Verification items for this drawing (mm, ordinates from the low corner). Round coordinates to 2 decimals unless told otherwise and drop trailing zeros. Loops run counter-clockwise (first coordinate to the right, second up) from the corner with the lowest first, then second, coordinate; pieces in that order, holes last. Notation, with made-up numbers: M -9,14.25 L 49,14.25 A14 ccw 49,37.25 Z; hole C -19.75,58.25 d11. An arc over 180 degrees is marked long. Write item = value, one per line. Start each with the question number.
(1) Scan lines: L1, parallel to X at y = 2, z = 51.5; L2, parallel to Z at x = 3, y = 7.25; L3, parallel to X at y = 3, z = 37. Record each from-to range of solid material in increasing order. Write a range as from..to.
(2) Cross-section at D-D on z = 28. Record the boundary of the cut face in (x, y), plus the area to 3 significant figures.
(3) Cross-section at B-B on x = 51.5. Record the boundary of the cut face in (y, z), plus the area to 3 significant figures.
(4) Cross-section at A-A on z = 4.5. Record the boundary of the cut face in (x, y).
(5) Cross-section at C-C on y = 5.25. Record the boundary of the cut face in (x, z), plus the area to 3 significant figures.
(6) Mould release check, pull along X, two halves, no side actions. Record for the marked faces 1, 2, 3 and 4: pulls with the +X half, pulls with the -X half, needs draft (parallel to the pull), parting line crosses it, or undercut.
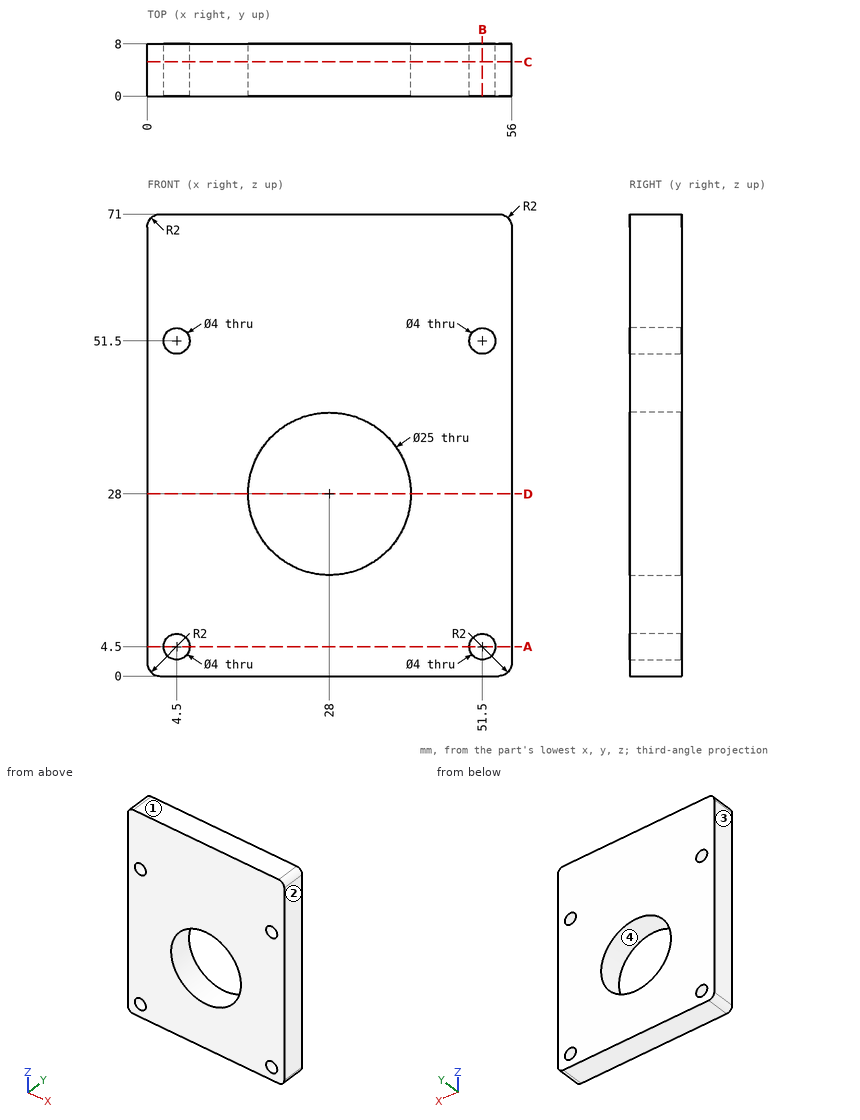
Result:
q1.L1 = 0..2.5, 6.5..49.5, 53.5..56
q1.L2 = 0..3.18, 5.82..50.18, 52.82..71
q1.L3 = 0..19.33, 36.67..56
q2.outline = M 0,0 L 15.5,0 L 15.5,8 L 0,8 Z; M 40.5,0 L 56,0 L 56,8 L 40.5,8 Z
q2.area = 248 mm^2
q3.outline = M 0,0 L 8,0 L 8,2.5 L 0,2.5 Z; M 0,6.5 L 8,6.5 L 8,49.5 L 0,49.5 Z; M 0,53.5 L 8,53.5 L 8,71 L 0,71 Z
q3.area = 504 mm^2
q4.outline = M 0,0 L 2.5,0 L 2.5,8 L 0,8 Z; M 6.5,0 L 49.5,0 L 49.5,8 L 6.5,8 Z; M 53.5,0 L 56,0 L 56,8 L 53.5,8 Z
q5.outline = M 0,2 A2 ccw 2,0 L 54,0 A2 ccw 56,2 L 56,69 A2 ccw 54,71 L 2,71 A2 ccw 0,69 Z; hole C 4.5,4.5 d4; hole C 4.5,51.5 d4; hole C 28,28 d25; hole C 51.5,4.5 d4; hole C 51.5,51.5 d4
q5.area = 3,430 mm^2
q6.face_1 = needs draft
q6.face_2 = pulls with the +X half
q6.face_3 = pulls with the -X half
q6.face_4 = undercut
